from build123d import *

# Parameters (mm, degrees)
BOSS_EXTRUDE1_DEPTH     = 2.54
CUT_EXTRUDE1_DEPTH      = 1
CUT_EXTRUDE1_DEPTH_BACK = 3.54


with BuildPart() as part:
    # Sketch1 → Boss-Extrude1 (new body)
    with BuildSketch(Plane.XY):
        Polygon((-945.957227657, 86.137779906), (-945.969713578, 86.1172966), (-949.121092485, 86.403457059), (-949.65244679, 80.075727402), (-9.887238192, -5.25964904), (-6.723373364, -5.525326193), (0, -5.833733414), (152.4, -5.833733414), (152.4, 11.946266586), (139.7, 11.946266586), (139.7, 6.866266586), (136.525, 6.866266586), (136.525, 11.946266586), (95.25, 11.946266586), (95.25, 6.866266586), (92.075, 6.866266586), (92.075, 11.946266586), (79.375, 11.946266586), (79.375, 6.866266586), (76.2, 6.866266586), (76.2, 11.946266586), (69.85, 11.946266586), (25.4, 19.566266586), (19.05, 19.566266586), (19.05, 14.486266586), (15.875, 14.486266586), (15.875, 19.566266586), (3.175, 19.566266586), (3.175, 13.216266586), (0, 13.216266586), (0, 19.566266586), (-1.98607431, 19.566266586), (-4.597956143, 19.785592432), (-5.129310448, 13.457862776), (-8.293175277, 13.723539928), (-7.761820971, 20.051269584), (-944.89858306, 98.744842179), align=None)
    extrude(amount=BOSS_EXTRUDE1_DEPTH)

    # Sketch2 → Cut-Extrude1 (cut, two sides)
    with BuildSketch(Plane.XY.offset(2.54)) as cut_extrude1_sk:
        Polygon((-77.240292597, 25.885539855), (-80.404157425, 26.151217008), (-80.935453586, 19.824179771), (-77.77159129, 19.55847246), align=None)
        Polygon((-156.741594191, 26.190526923), (-156.210358707, 32.516841584), (-159.374223535, 32.782518736), (-159.905456487, 26.456234233), align=None)
        Polygon((-235.711597092, 32.822581386), (-235.180424816, 39.148143312), (-238.344289645, 39.413820465), (-238.875459388, 33.088288696), align=None)
        Polygon((-314.681599993, 39.454635849), (-314.150490926, 45.77944504), (-317.314355754, 46.045122193), (-317.845462289, 39.720343159), align=None)
        Polygon((-393.651602894, 46.086690311), (-393.120557036, 52.410746769), (-396.284421864, 52.676423921), (-396.81546519, 46.352397622), align=None)
        Polygon((-472.621605795, 52.718744774), (-472.090623146, 59.042048497), (-475.254487974, 59.30772565), (-475.785468091, 52.984452084), align=None)
        Polygon((-551.591608696, 59.350799237), (-551.060689256, 65.673350226), (-554.224554084, 65.939027378), (-554.755470992, 59.616506547), align=None)
        Polygon((-630.561611597, 65.9828537), (-630.030755365, 72.304651954), (-633.194620194, 72.570329107), (-633.725473893, 66.24856101), align=None)
        Polygon((-709.531614498, 72.614908162), (-709.000821475, 78.935953682), (-712.164686303, 79.201630835), (-712.695476794, 72.880615473), align=None)
        Polygon((-788.501617399, 79.246962625), (-787.970887585, 85.567255411), (-791.134752413, 85.832932563), (-791.665479694, 79.512669935), align=None)
        Polygon((-867.4716203, 85.879017088), (-866.940953695, 92.198557139), (-870.104818523, 92.464234292), (-870.635482595, 86.144724398), align=None)
    extrude(amount=CUT_EXTRUDE1_DEPTH, mode=Mode.SUBTRACT)
    extrude(cut_extrude1_sk.sketch, amount=-CUT_EXTRUDE1_DEPTH_BACK, mode=Mode.SUBTRACT)


solid = part.part
Model file for the job. Use its own axes, mm. Give positions to 0.01 mm unless a question says otherwise; leave off trailing zeros. Loops run counter-clockwise (first coordinate to the right, second up) from the corner with the lowest first, then second, coordinate; pieces in that order, holes last.
1) Flat gauge pins, fed straight in: pin 1 Ø0.8 at (x, z) = (94.5, 2) entering from +Y; pin 2 Ø0.8 at (x, z) = (22, 1) entering from +Y. Where does each tip first touch, or does it go through?
2) Saw through at B-B (x = -444). Write the cut outline in (y, z), plus the area to 3 significant figures.
3) Saw through at A-A (x = -264.5). Write the cut outline in (y, z).
4) Wall check: line 1 (Y direction, x = 63, z = 1.05); line 2 (Y direction, x = -790, z = 0.6). Give the ranges that are in metal, low to high.
Answer block:
1. pin 1: stops at y = 6.87
1. pin 2: stops at y = 19.57
2. outline: (34.16, 0) - (56.68, 0) - (56.68, 2.54) - (34.16, 2.54) - close
2. area: 57.2 mm2
3. outline: (17.86, 0) - (41.61, 0) - (41.61, 2.54) - (17.86, 2.54) - close
4. line 1: y = -5.83 to 13.12
4. line 2: y = 65.58 to 79.37
